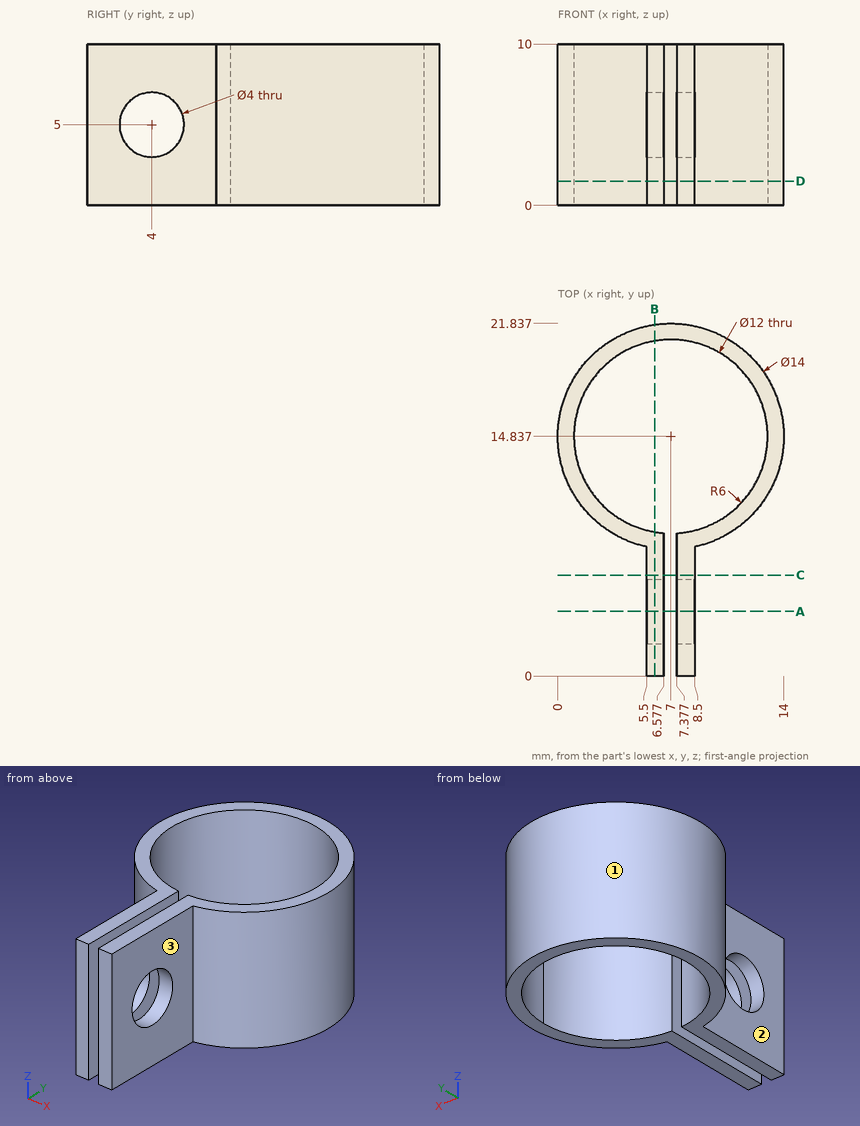
The drawing under review shows one solid part. Ordinate dimensions are in mm from its lowest x, y, z. A direction names the side the tool comes from. Coordinates: 2 decimals unless noted, no trailing zeros. Order: outer loops, then holes, each group sorted by start corner. A loop starts at its lowest first (then second) coordinate and runs counter-clockwise, first axis right, second up. Notation, with made-up numbers: (59.25, 19.25) -> (103.25, 19.25) arc R8 ccw to (103.25, 32.25) -> close; hole circle Ø10 at (-0.5, 25). An arc over 180 degrees is marked (long way). Return JSON: item names as keys, results as strings.
1. For line 1 (X direction, y = 1.5, z = 7.25); line 2 (Y direction, x = 5.8, z = 5); line 3 (Y direction, x = 6.25, z = 5) (1 decimal), list the stretches that pass through material, from the lowest coordinate up. Write a range as from..to.
Answer block:
{"line 1": "5.5..6.58, 7.38..8.5", "line 2": "0..2, 6..8.96, 20.72..21.73", "line 3": "0..2, 6..8.9, 20.8..21.8"}
2. For pin 1 Ø2.5 at (y, z) = (3, 6) entering from -X; pin 2 Ø2 at (x, z) = (5.5, 3) entering from -Y; pin 3 Ø1 at (x, z) = (6, 1.5) entering from +Y; pin 4 Ø2.5 at (y, z) = (4.5, 6.5) entering from +X, all flat-tipped, find the tip position at first contact; note any pin that passes through.
Answer block:
{"pin 1": "x = 5.5", "pin 2": "y = 0", "pin 3": "y = 21.82", "pin 4": "x = 8.5"}
3. We need section C-C on y = 6.25. Write out the cut boundary in (x, z), and give its area (3 significant figures).
Answer block:
{"outline": "(5.5, 0) -> (6.58, 0) -> (6.58, 10) -> (5.5, 10) -> close; (7.38, 0) -> (8.5, 0) -> (8.5, 10) -> (7.38, 10) -> close", "area": "22.0 mm²"}
4. We need section A-A on y = 4. Write out the cut boundary in (x, z).
Answer block:
{"outline": "(5.5, 0) -> (6.58, 0) -> (6.58, 3) -> (5.5, 3) -> close; (5.5, 7) -> (6.58, 7) -> (6.58, 10) -> (5.5, 10) -> close; (7.38, 0) -> (8.5, 0) -> (8.5, 3) -> (7.38, 3) -> close; (7.38, 7) -> (8.5, 7) -> (8.5, 10) -> (7.38, 10) -> close"}
5. Machinability: for the marked faces 1, 2 and 3, which of the approach directions +Z, -Z, +X, -X, +Y, -Y give a long, thin tool a straight path to every point of the face, cutting with its end or side? Answer none if there is none.
Answer block:
{"face 1": "+Z, -Z", "face 2": "+Z, -Z, -X, -Y", "face 3": "+Z, -Z, +X, -Y"}
6. We need section D-D on z = 1.5. Write out the cut boundary in (x, y).
Answer block:
{"outline": "(5.5, 0) -> (6.58, 0) -> (6.58, 8.85) arc R6 cw (long way) to (7.38, 8.85) -> (7.38, 0) -> (8.5, 0) -> (8.5, 8) arc R7 ccw (long way) to (5.5, 8) -> close"}
7. We need section B-B on x = 6. Write out the cut boundary in (y, z) (1 decimal).
Answer block:
{"outline": "(0, 0) -> (8.9, 0) -> (8.9, 10) -> (0, 10) -> close; (20.8, 0) -> (21.8, 0) -> (21.8, 10) -> (20.8, 10) -> close; hole circle Ø4 at (4, 5)"}
